Verification items for this drawing (mm, ordinates from the low corner). Coordinates: 2 decimals unless noted, no trailing zeros. Order: outer loops, then holes, each group sorted by start corner. A loop starts at its lowest first (then second) coordinate and runs counter-clockwise, first axis right, second up. Notation, with made-up numbers: M -38.5,78 L -34.5,78 A34 cw -34.5,111 Z; hole C 37.25,7 d2. An arc over 180 degrees is marked long. Return JSON: item names as keys, results as strings. Group by question number.
1. Material ranges on line 1 along X through (y, z) = (12.25, 2.75) (1 decimal); line 2 along X through (y, z) = (11.25, 15.75) (1 decimal); line 3 along Y through (x, z) = (12.75, 12.5) (1 decimal), recorded low to high.
2. Section check B-B, the plane y = 7.25. Record the cut outline in (x, z) (1 decimal), plus the area to 3 significant figures.
3. Section check A-A, the plane x = 7.25. Record the cut outline in (y, z) (1 decimal).
4. Section check D-D, the plane y = 18.25. Record the cut outline in (x, z).
5. Mould release check, pull along X, two halves, no side actions. Record for the marked faces 1, 2 and 3: +X half, -X half, draft (parallel to the pull), parting line (faces both ways), or undercut.
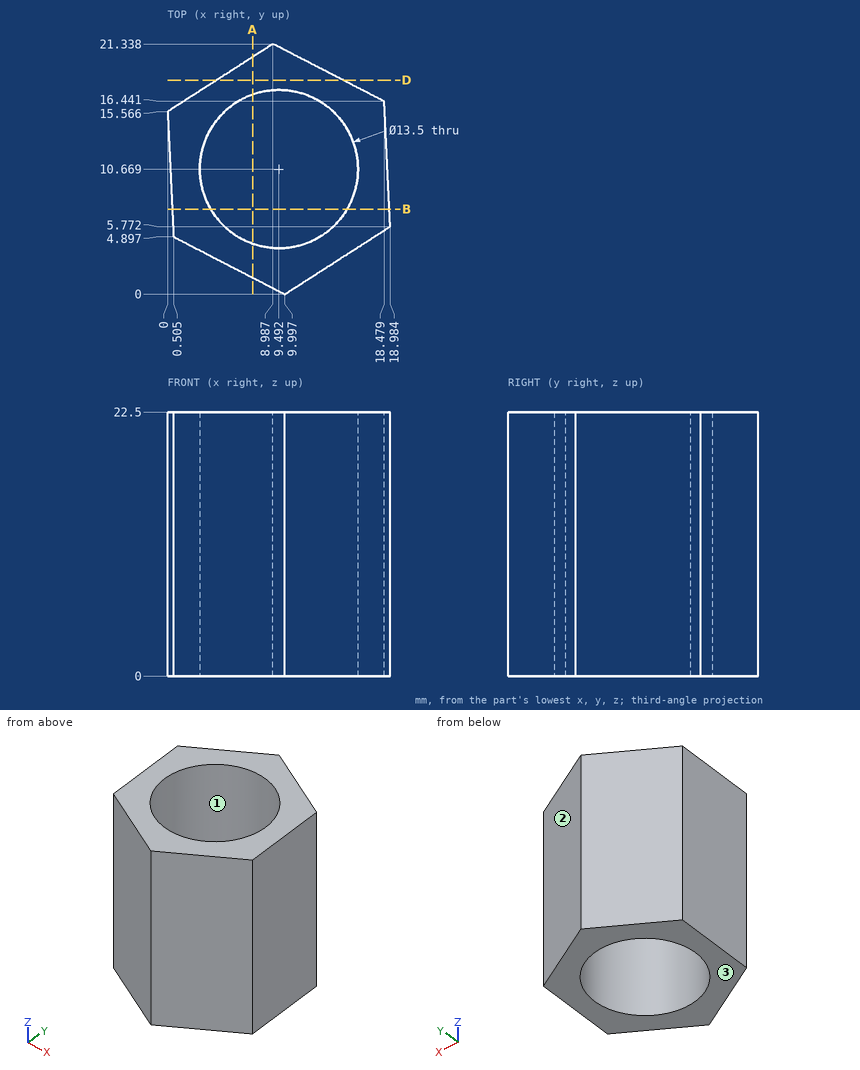
Answers follow:
{
 "1": {"line 1": "0.2 to 2.9, 16.1 to 18.7", "line 2": "0.2 to 2.8, 16.2 to 18.7", "line 3": "1.8 to 4.8, 16.6 to 19.4"},
 "2": {"outline": "M 0.4,0 L 3.7,0 L 3.7,22.5 L 0.4,22.5 Z; M 15.3,0 L 18.9,0 L 18.9,22.5 L 15.3,22.5 Z", "area": "155 mm^2"},
 "3": {"outline": "M 1.4,0 L 4.3,0 L 4.3,22.5 L 1.4,22.5 Z; M 17,0 L 20.2,0 L 20.2,22.5 L 17,22.5 Z"},
 "4": {"outline": "M 4.18,0 L 14.97,0 L 14.97,22.5 L 4.18,22.5 Z"},
 "5": {"face 1": "undercut", "face 2": "+X half", "face 3": "draft"}
}
